```python
from build123d import *

# Parameters (mm, degrees)
F0_R     = 12.7625
F0_R_2   = 6.4125
F1_DEPTH = 1.793748
F2_R     = 11.175
F2_R_2   = 6.4125
F3_DEPTH = 8
F4_R     = 12.7625
F4_R_2   = 6.4125
F5_DEPTH = 1.793748
F6_R     = 8
F7_DEPTH = 5
F8_R     = 8
F9_DEPTH = 5


with BuildPart() as f1:
    # F0 (on Top) → F1 (new body)
    with BuildSketch(Plane.XY):
        Circle(F0_R)
        Circle(F0_R_2, mode=Mode.SUBTRACT)
    extrude(amount=F1_DEPTH)

    # F2 (on face) → F3 (join)
    with BuildSketch(Plane.XY.offset(1.793748)):
        Circle(F2_R)
        Circle(F2_R_2, mode=Mode.SUBTRACT)
    extrude(amount=F3_DEPTH)

    # F4 (on face) → F5 (join)
    with BuildSketch(Plane.XY.offset(9.793748)):
        Circle(F4_R)
        Circle(F4_R_2, mode=Mode.SUBTRACT)
    extrude(amount=F5_DEPTH)

    # F6 (on face) → F7 (cut)
    with BuildSketch(Plane(origin=(0, 0, 0), x_dir=(1, 0, 0), z_dir=(0, 0, -1))):
        Circle(F6_R)
    extrude(amount=-F7_DEPTH, mode=Mode.SUBTRACT)

    # F8 (on face) → F9 (cut)
    with BuildSketch(Plane.XY.offset(11.587496)):
        Circle(F8_R)
    extrude(amount=-F9_DEPTH, mode=Mode.SUBTRACT)


solid = f1.part
```
Can you work these out from the model? Positions are in its coordinate system, mm. A direction names the side the tool comes from. Round coordinates to 2 decimals unless told otherwise and drop trailing zeros. Loops run counter-clockwise (first coordinate to the right, second up) from the corner with the lowest first, then second, coordinate; pieces in that order, holes last. Notation, with made-up numbers: (9.25, 86) -> (29.25, 86) arc R15 ccw to (29.25, 106) -> close; hole circle Ø6 at (39, 7). An arc over 180 degrees is marked (long way). Answer in a Markdown table with one row per item.
Item 1: Will these pins go through, and if not, where does the flat tip stop? P1, Ø3, axis at y = 2.5, z = 2.5, coming from the +X side; P2, Ø6, axis at x = 1.5, y = 5.5, coming from the -Z side; P3, Ø4, axis at x = 9, z = 9.5, coming from the +Y side; P4, Ø9.5, axis at x = 0, y = 0, coming from the +Z side.
Answer block:
| item | result |
|---|---|
| P1 | x = 12.71 |
| P2 | z = 0 |
| P3 | y = 10.66 |
| P4 | through |
Item 2: On a 3-axis mill with a long thin cutter (end or side, diameter ignored), from which of +Z, -Z, +X, -X, +Y, -Y can I reach the whole of each face in a straight line? I mean faces 4 (the flat face through (-0.2, -8.3, 0)), 5 (the cylindrical face through (-1.73, -7.81, 9.12)), 6 (the cylindrical face through (-1.45, 11.08, 5.74)), 7 (the cylindrical face through (-1.73, 7.81, 2.46)). Say none if no direction works.
Answer block:
| item | result |
|---|---|
| face 4 | -Z, +X, -X, +Y, -Y |
| face 5 | +Z |
| face 6 | none |
| face 7 | -Z |
Item 3: Suppose I cut it at C-C, the plane z = 10.75. List the corners of the cut face in (x, y) for me (1 decimal).
Answer block:
| item | result |
|---|---|
| outline | circle Ø25.5 at (0, 0); hole circle Ø16 at (0, 0) |
Item 4: If I drill on probe 1 along Y at (x, z) = (0, 5.8) (1 decimal); probe 2 along Y at (x, z) = (0, 9.7) (3 decimals); probe 3 along Z at (x, y) = (-9.75, -6), over which ranges is the centre line in solid material (lowest first)?
Answer block:
| item | result |
|---|---|
| probe 1 | -11.2 to -6.4, 6.4 to 11.2 |
| probe 2 | -11.175 to -8, 8 to 11.175 |
| probe 3 | 0 to 1.79, 9.79 to 11.59 |
Item 5: We'd pull the mould along X, two halves only. Please class faces 1 (the cylindrical face through (-1.661, 12.654, 0.884)), 2 (the flat face through (0.9, -11.3, 9.794)), 3 (the flat face through (0, -7, 5)): released by +X, released by -X, zero draft, split by the parting line, or undercut.
Answer block:
| item | result |
|---|---|
| face 1 | split by the parting line |
| face 2 | zero draft |
| face 3 | undercut |
Item 6: Suppose I cut it at A-A, the plane y = 0. List the corners of the cut face in (x, z) for me (1 decimal).
Answer block:
| item | result |
|---|---|
| outline | (-12.8, 0) -> (-8, 0) -> (-8, 5) -> (-6.4, 5) -> (-6.4, 6.6) -> (-8, 6.6) -> (-8, 11.6) -> (-12.8, 11.6) -> (-12.8, 9.8) -> (-11.2, 9.8) -> (-11.2, 1.8) -> (-12.8, 1.8) -> close; (6.4, 5) -> (8, 5) -> (8, 0) -> (12.8, 0) -> (12.8, 1.8) -> (11.2, 1.8) -> (11.2, 9.8) -> (12.8, 9.8) -> (12.8, 11.6) -> (8, 11.6) -> (8, 6.6) -> (6.4, 6.6) -> close |
Item 7: Suppose I cut it at D-D, the plane x = -10.5. List the corners of the cut face in (y, z) for me (1 decimal).
Answer block:
| item | result |
|---|---|
| outline | (-7.3, 0) -> (7.3, 0) -> (7.3, 1.8) -> (3.8, 1.8) -> (3.8, 9.8) -> (7.3, 9.8) -> (7.3, 11.6) -> (-7.3, 11.6) -> (-7.3, 9.8) -> (-3.8, 9.8) -> (-3.8, 1.8) -> (-7.3, 1.8) -> close |
